from build123d import *

# Parameters (mm, degrees)
SKETCH_W     = 70
SKETCH_H     = 60
SKETCH_W_2   = 15
SKETCH_H_2   = 3
PAD_DEPTH    = 2
SKETCH001_W  = 2
SKETCH001_H  = 15
POCKET_DEPTH = 2


with BuildPart() as part:
    # Sketch → Pad (new body)
    with BuildSketch(Plane.XY):
        with Locations((35, 30)):
            Rectangle(SKETCH_W, SKETCH_H)
        with Locations((35, 61.5)):
            Rectangle(SKETCH_W_2, SKETCH_H_2)
        with Locations((35, -1.5)):
            Rectangle(SKETCH_W_2, SKETCH_H_2)
    extrude(amount=PAD_DEPTH)

    # Sketch001 → Pocket (cut)
    with BuildSketch(Plane.XY):
        with Locations((66, 30)):
            Rectangle(SKETCH001_W, SKETCH001_H)
        with Locations((4, 30)):
            Rectangle(SKETCH001_W, SKETCH001_H)
    extrude(amount=POCKET_DEPTH, mode=Mode.SUBTRACT)


solid = part.part
Can you work these out from the model? Positions are in its coordinate system, mm. A direction names the side the tool comes from. Coordinates: 2 decimals unless noted, no trailing zeros. Write each loop counter-clockwise with the first axis right and the second up, starting at its lowest first coordinate (ties: lowest second). Pieces come first, ordered by that corner, then holes. Notation, with made-up numbers: M 67.25,24.5 L 108.25,24.5 A27 cw 108.25,59.5 Z; hole C 70.5,31.5 d10. An arc over 180 degrees is marked long. Use one line per item in the form item = value.
Q1. If we section it at B-B (z = 0.6): Write out the boundary of the cut face in (x, y), then the cut area to 3 significant figures.
Model answer:
outline = M 0,0 L 27.5,0 L 27.5,-3 L 42.5,-3 L 42.5,0 L 70,0 L 70,60 L 42.5,60 L 42.5,63 L 27.5,63 L 27.5,60 L 0,60 Z; hole M 3,22.5 L 5,22.5 L 5,37.5 L 3,37.5 Z; hole M 65,22.5 L 67,22.5 L 67,37.5 L 65,37.5 Z
area = 4,230 mm^2
Q2. If we section it at C-C (x = 58): Write out the boundary of the cut face in (y, z), then the cut area to 3 significant figures.
Model answer:
outline = M 0,0 L 60,0 L 60,2 L 0,2 Z
area = 120 mm^2
Q3. We'd pull the mould along X, two halves only. Please class faces 1 (the flat face through (42.5, 61, 1)), 2 (the flat face through (56, 60, 1)), 3 (the flat face through (65, 30, 1)): +X half, -X half, draft (parallel to the pull), parting line (faces both ways), or undercut.
Model answer:
face_1 = +X half
face_2 = draft
face_3 = undercut
Q4. I need wall thicknesses on line 1 along X through (y, z) = (26, 1.2); line 2 along Y through (x, z) = (45.5, 1.45); line 3 along X through (y, z) = (60.5, 0.15). Which ranges of each line are inside material? Lowest first, please. Write a range as from..to.
Model answer:
line_1 = 0..3, 5..65, 67..70
line_2 = 0..60
line_3 = 27.5..42.5
Q5. If we section it at A-A (y = 26): Write out the boundary of the cut face in (x, z), then the cut area to 3 significant figures.
Model answer:
outline = M 0,0 L 3,0 L 3,2 L 0,2 Z; M 5,0 L 65,0 L 65,2 L 5,2 Z; M 67,0 L 70,0 L 70,2 L 67,2 Z
area = 132 mm^2
Q6. For faces 4 (the flat face through (14, 60, 1)), 5 (the flat face through (3, 30, 1)), 6 (the flat face through (42.5, -2, 1)), 7 (the flat face through (27.5, -2, 1)), which set-ups out of +Z, -Z, +X, -X, +Y, -Y let a thin tool reach every point of the face, with its end or its side?
Model answer:
face_4 = +Z, -Z, -X, +Y
face_5 = +Z, -Z
face_6 = +Z, -Z, +X, -Y
face_7 = +Z, -Z, -X, -Y
Q7. For P1, Ø0.6, axis at x = 7.5, z = 1, coming from the +Y side; P2, Ø0.6, axis at x = 16.5, z = 1.5, coming from the -Y side; P3, Ø0.6, axis at y = 61.5, z = 1, coming from the +X side, each with a flat end and sliding along its axis, tell me the tip position at first contact or that it passes through.
Model answer:
P1 = 60
P2 = 0
P3 = 42.5
